Part model, mm, in its own coordinate system. Face numbers are marked on the shaded views. A direction names the side the tool comes from. Round coordinates to 2 decimals unless told otherwise and drop trailing zeros. Order: outer loops, then holes, each group sorted by start corner. A loop starts at its lowest first (then second) coordinate and runs counter-clockwise, first axis right, second up. Notation, with made-up numbers: (70, 75) - (115, 75) arc R12 ccw to (115, 84) - close; hole circle Ø1 at (-14.75, 69). An arc over 180 degrees is marked (long way). Answer as a JSON object with one key per item and string values.
```python
from build123d import *

# Parameters (mm, degrees)
SKETCH1_R           = 4.425
SKETCH1_R_2         = 2
SKETCH1_R_3         = 4
BOSS_EXTRUDE1_DEPTH = 3
SKETCH1_3_R         = 4
SKETCH1_3_R_2       = 2
BOSS_EXTRUDE2_DEPTH = 8
BOSS_EXTRUDE3_DEPTH = 11


with BuildPart() as part:
    # Sketch1 → Boss-Extrude1 (new body)
    with BuildSketch(Plane(origin=(0, 0, 0), x_dir=(1, 0, 0), z_dir=(0, 1, 0))):
        with BuildLine():
            ThreePointArc((1.322875656, 1.5), (0, 2), (-1.322875656, 1.5))
            Line((-1.322875656, 1.5), (1.322875656, 1.5))
        make_face()
        with BuildLine():
            Line((1.322875656, 1.5), (-1.322875656, 1.5))
            ThreePointArc((-1.322875656, 1.5), (-0.822875656, -1.822875656), (2, 0))
            ThreePointArc((2, 0), (1.822875656, 0.822875656), (1.322875656, 1.5))
        make_face()
        Circle(SKETCH1_R)
        Circle(SKETCH1_R_2, mode=Mode.SUBTRACT)
        Circle(SKETCH1_R)
        Circle(SKETCH1_R_3, mode=Mode.SUBTRACT)
    extrude(amount=BOSS_EXTRUDE1_DEPTH)

    # Sketch1<3> → Boss-Extrude2 (add)
    with BuildSketch(Plane(origin=(0, 0, 0), x_dir=(1, 0, 0), z_dir=(0, 1, 0))):
        Circle(SKETCH1_3_R)
        Circle(SKETCH1_3_R_2, mode=Mode.SUBTRACT)
        with BuildLine():
            ThreePointArc((1.322875656, 1.5), (0, 2), (-1.322875656, 1.5))
            Line((-1.322875656, 1.5), (1.322875656, 1.5))
        make_face()
        with BuildLine():
            Line((1.322875656, 1.5), (-1.322875656, 1.5))
            ThreePointArc((-1.322875656, 1.5), (-0.822875656, -1.822875656), (2, 0))
            ThreePointArc((2, 0), (1.822875656, 0.822875656), (1.322875656, 1.5))
        make_face()
    extrude(amount=BOSS_EXTRUDE2_DEPTH)

    # Sketch1<4> → Boss-Extrude3 (add)
    with BuildSketch(Plane(origin=(0, 0, 0), x_dir=(1, 0, 0), z_dir=(0, 1, 0))):
        with BuildLine():
            Line((1.322875656, 1.5), (-1.322875656, 1.5))
            ThreePointArc((-1.322875656, 1.5), (-0.822875656, -1.822875656), (2, 0))
            ThreePointArc((2, 0), (1.822875656, 0.822875656), (1.322875656, 1.5))
        make_face()
    extrude(amount=-BOSS_EXTRUDE3_DEPTH)


solid = part.part
```
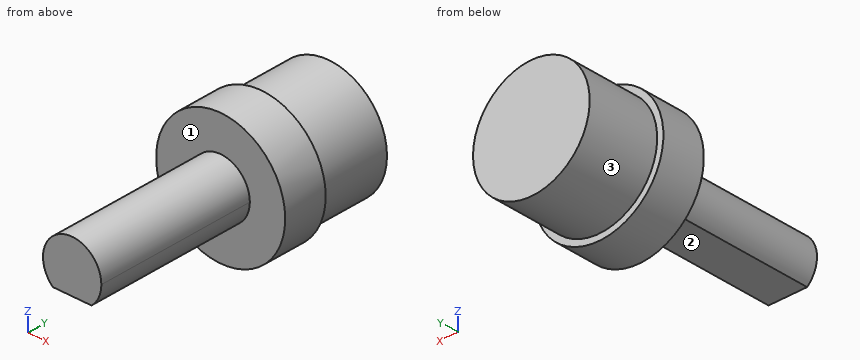
Item 1: Probe L1, parallel to Y at x = 2.25, z = 2.25; L2, parallel to Y at x = -3.75, z = 2.25; L3, parallel to X at y = -1.25, z = -0.25. List the from-to ranges inside material, lowest first. Write a range as from..to.
Taken from the geometry:
{"L1": "0..8", "L2": "0..3", "L3": "-1.98..1.98"}
Item 2: Drop flat-ended pins along their axis: P1, Ø1.3, axis at x = -0.5, y = -3, coming from the -Z side; P2, Ø5, axis at x = -2, z = 1.5, coming from the -Y side; P3, Ø3, axis at x = 3.5, z = 0.5, coming from the -Y side; P4, Ø2, axis at y = 4, z = 3.5, coming from the +X side. Give the stop position or say it passes through.
Taken from the geometry:
{"P1": "z = -1.5", "P2": "y = -11", "P3": "y = 0", "P4": "x = 3.12"}
Item 3: Cut at A-A (z = 2.75). Write the cut outline in (x, y).
Taken from the geometry:
{"outline": "(-3.47, 0) - (3.47, 0) - (3.47, 3) - (2.9, 3) - (2.9, 8) - (-2.9, 8) - (-2.9, 3) - (-3.47, 3) - close"}
Item 4: Cut at C-C (y = -7.5). Write the cut outline in (x, z), plus the area to 3 significant figures.
Taken from the geometry:
{"outline": "(-1.32, -1.5) - (1.32, -1.5) arc R2 ccw (long way) to start", "area": "11.7 mm2"}
Item 5: Tool access for the marked faces 1, 2 and 3: list every direction of +Z, -Z, +X, -X, +Y, -Y with a clear straight run to the whole face (end or side of a thin tool).
Taken from the geometry:
{"face 1": "-Y", "face 2": "-Z, +X, -X, -Y", "face 3": "+Y"}
Item 6: Cut at B-B (x = 0). Write the cut outline in (y, z) (3 decimals).
Taken from the geometry:
{"outline": "(-11, -1.5) - (0, -1.5) - (0, -4.425) - (3, -4.425) - (3, -4) - (8, -4) - (8, 4) - (3, 4) - (3, 4.425) - (0, 4.425) - (0, 2) - (-11, 2) - close"}
Item 7: Cut at D-D (z = -3.5). Write the cut outline in (x, y), plus the area to 3 significant figures.
Taken from the geometry:
{"outline": "(-2.71, 0) - (2.71, 0) - (2.71, 3) - (1.94, 3) - (1.94, 8) - (-1.94, 8) - (-1.94, 3) - (-2.71, 3) - close", "area": "35.6 mm2"}
